Read the model definition and answer for the solid it produces. Units are mm, in the model's axes. Round coordinates to 2 decimals unless told otherwise and drop trailing zeros. Write each loop counter-clockwise with the first axis right and the second up, starting at its lowest first coordinate (ties: lowest second). Pieces come first, ordered by that corner, then holes.
Autodesk Fusion 360 part; units mm, degrees
sketch "Sketch1" plane through (0, 0, 0) normal (0, 0, 1) x (1, 0, 0)
  line L0 (12.5, -3) -> (-12.5, -3)
  line L1 (-12.5, -3) -> (-12.5, 3)
  line L2 (-12.5, 3) -> (12.5, 3)
  line L3 (12.5, 3) -> (12.5, -3)
  line L4 (12.5, -3) -> (-12.5, 3) construction
  line L5 (-12.5, -3) -> (12.5, 3) construction
  dimension "d1" = 6
  dimension "d2" = 25
extrude "Extrude1" add sketch "Sketch1" along normal blind 21.616
sketch "Sketch2" plane through (0, -3, 0) normal (0, -1, 0) x (1, 0, 0)
  line L0 (-12.5, 0) -> (12.5, 0)
  line L1 (12.5, 0) -> (12.5, 21.616)
  line L2 (12.5, 21.616) -> (-12.5, 21.616)
  line L3 (-12.5, 21.616) -> (-12.5, 0)
  circle A0 centre (0, 21.616) radius 12.5
  circle A1 centre (0, 21.616) radius 9.5
  dimension "d5" = 19
extrude "Extrude2" add sketch "Sketch2" against normal blind 6 contours L2 A0 A1 picked at (-11.4535, 22.237)
extrude "Extrude3" cut sketch "Sketch2" against normal blind 6 contours L2 A1 picked at (0.2366, 18.4582)
Q1. Section A-A (x = -3.75) is taken. Determine the outline of the cut face in (y, z).
Verdict:
outline: (-3, 0) - (3, 0) - (3, 12.89) - (-3, 12.89) - close; (-3, 30.34) - (3, 30.34) - (3, 33.54) - (-3, 33.54) - close
Q2. Section B-B (y = -1.35) is taken. Determine the outline of the cut face in (x, z).
Verdict:
outline: (-12.5, 0) - (12.5, 0) - (12.5, 21.62) arc R12.5 ccw to (-12.5, 21.62) - close; hole circle Ø19 at (0, 21.62)
Q3. Section C-C (z = 18) is taken. Determine the outline of the cut face in (x, y), then the cut area to 3 significant figures.
Verdict:
outline: (-12.5, -3) - (-8.78, -3) - (-8.78, 3) - (-12.5, 3) - close; (8.78, -3) - (12.5, -3) - (12.5, 3) - (8.78, 3) - close
area: 44.6 mm2
Q4. Flat-ended cylindrical pins translate along their axes: pin 1 Ø2 at (x, y) = (7, 1) entering from +Z; pin 2 Ø4 at (x, z) = (-6, 21.5) entering from -Y. Find the tip coordinate at first contact, or state that the pin passes through.
Verdict:
pin 1: stops at z = 32.58
pin 2: passes through
Q5. Straight lines are drawn through the part: probe 1 along Z at (x, y) = (0, -1.55); probe 2 along Z at (x, y) = (5, -0.75); probe 3 along X at (y, z) = (2.55, 27.5). For each, find the intervals that lie inside material, in ascending order.
Verdict:
probe 1: z = 0 to 12.12, 31.12 to 34.12
probe 2: z = 0 to 13.54, 29.69 to 33.07
probe 3: x = -11.03 to -7.46, 7.46 to 11.03
Q6. Determine the mould class of faces 1 (the flat face through (12.5, 0, 11)), 2 (the cylindrical face through (-2.06, -0.04, 12.34)), 3 (the cylindrical face through (0.275, -0.042, 34.113)), 4 (the flat face through (0, -3, 9)) for opening direction X: pulls with the +X half, pulls with the -X half, needs draft (parallel to the pull), parting line crosses it, or undercut.
Verdict:
face 1: pulls with the +X half
face 2: undercut
face 3: parting line crosses it
face 4: needs draft
Q7. Section D-D (x = -10) is taken. Determine the outline of the cut face in (y, z), then the cut area to 3 significant figures.
Verdict:
outline: (-3, 0) - (3, 0) - (3, 29.12) - (-3, 29.12) - close
area: 175 mm2
